```python
from build123d import *

# Parameters (mm, degrees)
F0_W     = 38.1
F0_H     = 38.1
F1_DEPTH = 19.05
F2_W     = 19.05
F2_H     = 19.05
F3_DEPTH = 19.05
F5_SIZE  = 0.0254
F4_W     = 19.05
F4_H     = 19.05
F6_DEPTH = 19.05


with BuildPart() as f1:
    # F0 (on Front) → F1 (new body)
    with BuildSketch(Plane.XZ):
        with Locations((19.05, 19.05)):
            Rectangle(F0_W, F0_H)
    extrude(amount=F1_DEPTH)

    # F2 (on face) → F3 (join)
    with BuildSketch(Plane.XZ.offset(19.05)):
        with Locations((9.525, 28.575)):
            Rectangle(F2_W, F2_H)
    extrude(amount=F3_DEPTH)

    # F5
    f5_edges = [f1.edges().sort_by_distance(p)[0] for p in [
        (19.05, -28.575, 19.05),
    ]]
    chamfer(f5_edges, length=F5_SIZE)

    # F4 (on face) → F6 (join)
    with BuildSketch(Plane.XZ.offset(19.05)):
        with Locations((28.575, 9.525)):
            Rectangle(F4_W, F4_H)
    extrude(amount=F6_DEPTH)


solid = f1.part
```
Can you work these out from the model? Positions are in its coordinate system, mm. A direction names the side the tool comes from. Give positions to 0.01 mm unless a question says otherwise; leave off trailing zeros. Loops run counter-clockwise (first coordinate to the right, second up) from the corner with the lowest first, then second, coordinate; pieces in that order, holes last. Notation, with made-up numbers: M 64,-29 L 70,-29 A5 cw 70,-24 Z; hole C -39,77.25 d11. An arc over 180 degrees is marked long. Use CSV: the item, a comma, the result in double quotes. Start each with the question number.
1. On a 3-axis mill with a long thin cutter (end or side, diameter ignored), from which of +Z, -Z, +X, -X, +Y, -Y can I reach the whole of each face in a straight line? I mean faces 1 (the face through (28, -28, 19.05)), 2 (the face through (23, -15, 0)), 3 (the face through (19.05, -28, 9)). Say none if no direction works.
2. Imagine slicing it at B-B, the plane z = 26. Write out the boundary of the cut face in (x, y).
3. Imagine slicing it at C-C, the plane x = 22. Write out the boundary of the cut face in (y, z).
4. For P1, Ø1, axis at x = 26.5, y = -24, coming from the +Z side; P2, Ø21, axis at y = -32.5, z = 6.5, coming from the -X side; P3, Ø1, axis at x = 32, z = 30, coming from the -Y side, each with a flat end and sliding along its axis, tell me the tip position at first contact or that it passes through.
5. If I drill on L1, parallel to Z at x = 22.5, y = -24; L2, parallel to Z at x = 12.5, y = -21, over which ranges is the centre line in solid material (lowest first)?
Response values:
1,face 1,"+Z, +X, -Y"
1,face 2,"-Z, +X, -X, +Y, -Y"
1,face 3,"-Z, -X, -Y"
2,outline,"M 0,-38.1 L 19.05,-38.1 L 19.05,-19.05 L 38.1,-19.05 L 38.1,0 L 0,0 Z"
3,outline,"M -38.1,0 L 0,0 L 0,38.1 L -19.05,38.1 L -19.05,19.05 L -38.1,19.05 Z"
4,P1,"z = 19.05"
4,P2,"x = 19.05"
4,P3,"y = -19.05"
5,L1,"0 to 19.05"
5,L2,"19.05 to 38.1"
